from build123d import *

# Parameters (mm, degrees)
F1_DEPTH = 25.4
F2_R     = 12.7
F4_DEPTH = 12.7
F5_R     = 6.35
F6_DEPTH = 25.4


with BuildPart() as f1:
    # F0 (on Front) → F1 (new body, symmetric)
    with BuildSketch(Plane.XZ):
        Polygon((-37.249966, 34.434151), (0, 0), (48.737777, 0), (48.737777, 12.7), (4.970752, 12.7), (-28.62911, 43.759968), align=None)
    extrude(amount=F1_DEPTH, both=True)

    # F2
    f2_edges = [f1.edges().sort_by_distance(p)[0] for p in [
        (4.970752, 0, 12.7),
    ]]
    fillet(f2_edges, radius=F2_R)

    # F3 (on Front) → F4 (join, symmetric)
    with BuildSketch(Plane.XZ):
        Polygon((4.970752, 12.7), (27.530322, 12.7), (-11.595107, 28.013606), align=None)
    extrude(amount=F4_DEPTH, both=True)

    # F5 (on face) → F6 (cut)
    with BuildSketch(Plane(origin=(8.620855, 0, 9.325816), x_dir=(0.734316, 0, -0.678808), z_dir=(0.678808, 0, 0.734316))):
        with Locations((-38.027416, -12.7)):
            Circle(F5_R)
        with Locations((-38.027416, 12.7)):
            Circle(F5_R)
    extrude(amount=-F6_DEPTH, mode=Mode.SUBTRACT)


solid = f1.part
Work out the finished part from the listing and answer in its coordinate system (mm). A direction names the side the tool comes from. Give positions to 0.01 mm unless a question says otherwise; leave off trailing zeros. Order: outer loops, then holes, each group sorted by start corner. A loop starts at its lowest first (then second) coordinate and runs counter-clockwise, first axis right, second up. Notation, with made-up numbers: (71, 34) - (106, 34) arc R25 ccw to (106, 56) - close; hole circle Ø11 at (27.25, -30.75). An arc over 180 degrees is marked (long way). Answer as CSV lines item,"result". Start each with the question number.
Q1. Given pin 1 Ø6 at (y, z) = (7, 35) entering from +X; pin 2 Ø2 at (y, z) = (14.5, 25.5) entering from +X; pin 3 Ø10 at (y, z) = (-11.5, 23.5) entering from -X; pin 4 Ø10 at (x, y) = (8.5, -18.5) entering from -Z, each flat-ended and moving along its own axis, determine where each tip first touches the part or whether it passes through.
Q2. The part is cut by section B-B (y = -14). Write down the section's boundary in (x, z), then the cut area to 3 significant figures.
Q3. The mould has two halves that part along Z. Classify faces 1 (the face through (24, 0, 0)), 2 (the face through (2, -25.4, 11)), 3 (the face through (-24.56, -18.9, 31.48)): +Z half, -Z half, draft (parallel to the pull), parting line (faces both ways), or undercut.
Q4. The part is cut by section A-A (y = -2.5). Write down the section's boundary in (x, z).
Q5. For faces 4 (the face through (6, -12.7, 18)), 5 (the face through (34, 0, 12.7)), 6 (the face through (5.25, 19.14, 13.6)), 7 (the face through (8.24, -0.18, 20.25)), determine the directions among +Z, -Z, +X, -X, +Y, -Y from which every point of the face is accessible in a straight line to the end or side of a thin tool.
Q6. The part is cut by section D-D (z = 17). Write down the section's boundary in (x, y), then the cut area to 3 significant figures.
Q7. Find the intervals of material crossed by L1, parallel to Y at x = -18.5, z = 31; L2, parallel to Z at x = 32.5, y = 7; L3, parallel to Z at x = -12, y = 12, in increasing order. Write a range as [from, to].
Q8. The part is cut by section C-C (x = 39). Write down the section's boundary in (y, z), then the cut area to 3 significant figures.
Check result:
1,pin 1,"stops at x = -15.91"
1,pin 2,"stops at x = -7.79"
1,pin 3,"stops at x = -26.59"
1,pin 4,"stops at z = 0"
2,outline,"(-37.25, 34.43) - (-32.49, 30.03) - (-23.87, 39.36) - (-28.63, 43.76) - close; (-23.36, 21.59) - (0, 0) - (48.74, 0) - (48.74, 12.7) - (9.94, 12.7) arc R12.7 cw to (1.32, 16.07) - (-14.74, 30.92) - close"
2,area,"1,050 mm²"
3,face 1,"-Z half"
3,face 2,"draft"
3,face 3,"undercut"
4,outline,"(-37.25, 34.43) - (0, 0) - (48.74, 0) - (48.74, 12.7) - (27.53, 12.7) - (-11.6, 28.01) - (-28.63, 43.76) - close"
5,face 4,"+Z, +X, -Y"
5,face 5,"+Z, +X"
5,face 6,"+Z, +X, +Y"
5,face 7,"+Z, +X, +Y, -Y"
6,outline,"(-18.39, -25.4) - (0.32, -25.4) - (0.32, -12.7) - (16.54, -12.7) - (16.54, 12.7) - (0.32, 12.7) - (0.32, 25.4) - (-18.39, 25.4) - close"
6,area,"1,360 mm²"
7,L1,"y = [-25.4, -18.06], [-7.34, 7.34], [18.06, 25.4]"
7,L2,"z = [0, 12.7]"
7,L3,"z = [11.09, 28.39]"
8,outline,"(-25.4, 0) - (25.4, 0) - (25.4, 12.7) - (-25.4, 12.7) - close"
8,area,"645 mm²"
